```python
from build123d import *

# Parameters (mm, degrees)
RESSALTO_EXTRUS_O1_DEPTH                       = 40
ESBO_O2_R                                      = 6.5
CORTE_EXTRUS_O1_DEPTH                          = 19
CHANFRO1_SIZE2                                 = 6.5
CHANFRO1_SIZE                                  = 4
ESBO_O3_R                                      = 2
CORTE_EXTRUS_O2_DEPTH                          = 59.307816613
RESSALTO_EXTRUS_O2_DEPTH                       = 14
BROCA_DE_ROSQUEAR_PARA_TARRAXA_DE_5_16_1_D     = 6.5278
BROCA_DE_ROSQUEAR_PARA_TARRAXA_DE_5_16_1_DEPTH = 13
BROCA_DE_ROSQUEAR_PARA_TARRAXA_DE_5_16_1_TIP   = 1.961148974


with BuildPart() as part:
    # Esboço1 → Ressalto-extrusão1 (new body)
    with BuildSketch(Plane.XY):
        Polygon((-11.864884923, 0), (14.135115077, 0), (14.135115077, 40), (-11.864884923, 40), (-11.864884923, 30), (-6.091382231, 20), (-11.864884923, 10), align=None)
    extrude(amount=-RESSALTO_EXTRUS_O1_DEPTH)

    # Esboço2 → Corte-extrusão1 (cut)
    with BuildSketch(Plane(origin=(14.135115077, 0, 0), x_dir=(0, 0, -1), z_dir=(1, 0, 0))):
        with Locations((20, 20)):
            Circle(ESBO_O2_R)
    extrude(amount=-CORTE_EXTRUS_O1_DEPTH, mode=Mode.SUBTRACT)

    # Chanfro1
    chanfro1_edges = [part.edges().sort_by_distance(p)[0] for p in [
        (-4.864884923, 20, -13.5),
    ]]
    chanfro1_side = [part.faces().sort_by_distance(p)[0] for p in [
        (-4.784884923, 20, -13.5),
    ]]
    chamfer(chanfro1_edges, length=CHANFRO1_SIZE - 0.0001, length2=CHANFRO1_SIZE2 - 0.0001, reference=chanfro1_side[0])  # a hair under: the kernel refuses the full size

    # Esboço3 → Corte-extrusão2 (cut, through all)
    with BuildSketch(Plane.XY):
        with Locations((7.135115077, 26.5)):
            Circle(ESBO_O3_R)
    extrude(amount=-CORTE_EXTRUS_O2_DEPTH, mode=Mode.SUBTRACT)

    # Esboço4 → Ressalto-extrusão2 (add)
    with BuildSketch(Plane.XZ):
        with BuildLine():
            Line((-1.864884923, -13), (4.135115077, -13))
            ThreePointArc((4.135115077, -13), (11.135115077, -20), (4.135115077, -27))
            Line((4.135115077, -27), (-1.864884923, -27))
            ThreePointArc((-1.864884923, -27), (-8.864884923, -20), (-1.864884923, -13))
        make_face()
    extrude(amount=RESSALTO_EXTRUS_O2_DEPTH)

    # Broca de rosquear para tarraxa de 5/16-181
    with Locations(Plane(origin=(0, -14, 0), x_dir=(-1, 0, 0), z_dir=(0, -1, 0))):
        with Locations((-1.135115077, 20)):
            Hole(BROCA_DE_ROSQUEAR_PARA_TARRAXA_DE_5_16_1_D / 2, depth=BROCA_DE_ROSQUEAR_PARA_TARRAXA_DE_5_16_1_DEPTH)
            with Locations((0, 0, -(BROCA_DE_ROSQUEAR_PARA_TARRAXA_DE_5_16_1_DEPTH + BROCA_DE_ROSQUEAR_PARA_TARRAXA_DE_5_16_1_TIP / 2))):  # 118° drill point
                Cone(0, BROCA_DE_ROSQUEAR_PARA_TARRAXA_DE_5_16_1_D / 2, BROCA_DE_ROSQUEAR_PARA_TARRAXA_DE_5_16_1_TIP, mode=Mode.SUBTRACT)


solid = part.part
```
Here's how the part is built. I have some questions about the finished solid (model axes, mm). A direction names the side the tool comes from. Coordinates: 2 decimals unless noted, no trailing zeros. Order: outer loops, then holes, each group sorted by start corner. A loop starts at its lowest first (then second) coordinate and runs counter-clockwise, first axis right, second up.
Item 1: Thinking about a two-plate mould opening in Z: for faces 1 (the face through (6.74, 13.655, -18.591)), 2 (the face through (-11.865, 35, -20)), 3 (the face through (1, -7, -13)), which applies, pulls with the +Z half, pulls with the -Z half, needs draft (parallel to the pull), parting line crosses it, or undercut?
Response values:
face 1: undercut
face 2: needs draft
face 3: pulls with the +Z half
Item 2: I'm going to push flat-ended pins straight in: pin 1 Ø5 at (x, y) = (2, -6.5) entering from -Z; pin 2 Ø5 at (x, y) = (1, -9.5) entering from +Z; pin 3 Ø13 at (x, z) = (4.5, -11) entering from -Y; pin 4 Ø2 at (y, z) = (15.5, -28) entering from -X. Where does each tip first touch, or does it pass through?
Response values:
pin 1: stops at z = -27
pin 2: stops at z = -13
pin 3: stops at y = -14
pin 4: stops at x = -9.27
Item 3: Which directions (+Z, -Z, +X, -X, +Y, -Y) give clear straight access to the entire face, cutting with the end or side of a thin tool? Please do faces 4 (the face through (-8.863, -6.902, -20.154)), 5 (the face through (-9.02, 25.07, -19.72)), 6 (the face through (11.133, -6.902, -19.846)), 7 (the face through (2.641, -7.409, -17.104)), 8 (the face through (1, -7, -27)).
Response values:
face 4: -X, -Y
face 5: +Z, -Z, -X
face 6: +X, -Y
face 7: -Y
face 8: -Z, +X, -X, -Y
Item 4: I need wall thicknesses on probe 1 along X at (y, z) = (-9.5, -20); probe 2 along Y at (x, z) = (12.5, -38); probe 3 along Z at (x, y) = (-0.25, 15). Which ranges of each line are inside material? Lowest first, please.
Response values:
probe 1: x = -8.86 to -2.13, 4.4 to 11.14
probe 2: y = 0 to 40
probe 3: z = -40 to -24.15, -15.85 to 0
Item 5: If we section it at C-C, the plane x = -4: List the corners of the cut face in (y, z) for me, then the cut area to 3 significant figures.
Response values:
outline: (-14, -26.67) - (0, -26.67) - (0, -40) - (40, -40) - (40, 0) - (0, 0) - (0, -13.33) - (-14, -13.33) - close; hole circle Ø2.81 at (20, -20)
area: 1,780 mm2
Item 6: If we section it at A-A, the plane x = 7: List the corners of the cut face in (y, z) for me.
Response values:
outline: (-14, -26.39) - (0, -26.39) - (0, -40) - (24.5, -40) - (24.5, -24.69) arc R6.5 cw (long way) to (24.5, -15.31) - (24.5, 0) - (0, 0) - (0, -13.61) - (-14, -13.61) - close; (28.5, -40) - (40, -40) - (40, 0) - (28.5, 0) - close
Item 7: If we section it at B-B, the plane x = 10: List the corners of the cut face in (y, z) for me, then the cut area to 3 significant figures.
Response values:
outline: (-14, -23.82) - (0, -23.82) - (0, -40) - (40, -40) - (40, 0) - (0, 0) - (0, -16.18) - (-14, -16.18) - close; hole circle Ø13 at (20, -20)
area: 1,570 mm2
